Work out the finished part from the listing and answer in its coordinate system (mm). Face numbers are marked on the shaded views. A direction names the side the tool comes from. Round coordinates to 2 decimals unless told otherwise and drop trailing zeros. Order: outer loops, then holes, each group sorted by start corner. A loop starts at its lowest first (then second) coordinate and runs counter-clockwise, first axis right, second up. Notation, with made-up numbers: M 33,15 L 47,15 A30 cw 47,45 Z; hole C 5,-20.75 d3. An arc over 180 degrees is marked long. Answer as a JSON object with one key per item and string values. Group by question number.
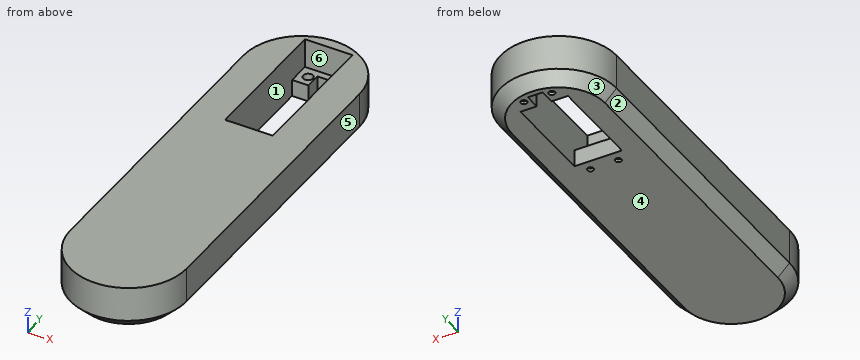
from build123d import *

# Parameters (mm, degrees)
BOSS_EXTRUDE1_DEPTH = 10
CHAMFER1_SIZE       = 5
CUT_EXTRUDE1_DEPTH  = 10.25
SKETCH5_W           = 6.4
SKETCH5_H           = 6.71
CUT_EXTRUDE2_DEPTH  = 24


with BuildPart() as part:
    # Sketch1 → Boss-Extrude1 (new, symmetric)
    with BuildSketch(Plane.XY):
        with BuildLine():
            Line((25, 130), (25, 0))
            ThreePointArc((25, 0), (0, -25), (-25, 0))
            Line((-25, 0), (-25, 130))
            ThreePointArc((-25, 130), (0, 155), (25, 130))
        make_face()
    extrude(amount=BOSS_EXTRUDE1_DEPTH, both=True)

    # Chamfer1
    chamfer1_edges = [part.edges().sort_by_distance(p)[0] for p in [
        (25, 65, -10),
        (0, -25, -10),
        (-25, 65, -10),
        (0, 155, -10),
    ]]
    chamfer(chamfer1_edges, length=CHAMFER1_SIZE)

    # Sketch3 → Cut-Extrude1 (cut, symmetric)
    with BuildSketch(Plane(origin=(0, 0, 0), x_dir=(0, 0, -1), z_dir=(1, 0, 0))):
        Polygon((2.7, 140.79), (2.7, 150.5), (-10, 150.5), (-10, 120.5), (10, 120.5), (10, 140.79), align=None)
    cut_extrude1 = extrude(amount=CUT_EXTRUDE1_DEPTH, both=True, mode=Mode.SUBTRACT)

    # Sketch4 → Cut-Revolve1 (revolve, cut)
    with BuildSketch(Plane(origin=(-6, 0, 0), x_dir=(0, 0, -1), z_dir=(1, 0, 0)), mode=Mode.PRIVATE) as cut_revolve1_sk:
        Polygon((2.7, 145.5), (12.7, 145.5), (12.7, 146.85), (8.7, 146.85), (8.7, 147.6), (2.7, 147.6), align=None)
    cut_revolve1 = revolve(cut_revolve1_sk.sketch.rotate(Axis((-6, 145.5, -58.145818423), (0, 0, 1)), 90), axis=Axis((-6, 145.5, -58.145818423), (0, 0, 1)), mode=Mode.SUBTRACT)

    # Mirror1: Cut-Revolve1 across plane
    add(cut_revolve1.mirror(Plane(origin=(0, 0, 0), x_dir=(0, 0, 1), z_dir=(1, 0, 0))), mode=Mode.SUBTRACT)

    # Mirror2: Cut-Extrude1, Cut-Revolve1 across plane
    add(cut_extrude1.mirror(Plane(origin=(-10.25, 120.5, -10), x_dir=(0, 0, 1), z_dir=(0, -1, 0))), mode=Mode.SUBTRACT)
    add(cut_revolve1.mirror(Plane(origin=(-10.25, 120.5, -10), x_dir=(0, 0, 1), z_dir=(0, -1, 0))), mode=Mode.SUBTRACT)

    # Mirror2 copy 1 sketch → Mirror2 copy 1 (revolve, cut)
    with BuildSketch(Plane(origin=(6, 241, 0), x_dir=(0, 0, -1), z_dir=(-1, 0, 0))):
        Polygon((2.7, 145.5), (12.7, 145.5), (12.7, 146.85), (8.7, 146.85), (8.7, 147.6), (2.7, 147.6), align=None)
    revolve(axis=Axis((6, 95.5, -58.145818423), (0, 0, 1)), mode=Mode.SUBTRACT)

    # Sketch5 → Cut-Extrude2 (cut)
    with BuildSketch(Plane.XY.offset(-2.7)):
        with Locations((0, 144.145)):
            Rectangle(SKETCH5_W, SKETCH5_H)
    extrude(amount=-CUT_EXTRUDE2_DEPTH, mode=Mode.SUBTRACT)


solid = part.part
Item 1: Each of these flat-tipped pins is pushed along its axis until it touches: pin 1 (8 mm diameter, centred on x = -4, z = -6, fed in from +Y); pin 2 (5.5 mm diameter, centred on x = 8, z = -7.5, fed in from -Y); pin 3 (5.5 mm diameter, centred on x = -7, z = -8, fed in from -Y). Where does it stop, or does it pass through?
Item 2: The mould has two halves that part along X. Classify the marked faces 3, 4, 5 and 6: +X half, -X half, draft (parallel to the pull), parting line (faces both ways), or undercut.
Item 3: Consider L1, parallel to X at y = 145.5, z = -5.7; L2, parallel to Y at x = -6, z = -9.2; L3, parallel to Y at x = -6, z = -6. Determine where each line is inside the solid, lowest interval first.
Item 4: Find section B-B (z = 7.5). Give the vertices of the cut face in (x, y).
Item 5: A tool of negligible diameter and unlimited length cuts with its end or side. For the marked faces 1 and 2, from which of +Z, -Z, +X, -X, +Y, -Y can it reach the whole face along a straight path? Write none if from no direction.
Item 6: Find section C-C (y = 29). Give the vertices of the cut face in (x, z).
Item 7: Find section A-A (x = 0). Give the vertices of the cut face in (y, z), and give its area (3 significant figures).
Responses:
{
 "1": {"pin 1": "stops at y = 155", "pin 2": "stops at y = -24.04", "pin 3": "stops at y = -23.84"},
 "2": {"face 3": "parting line", "face 4": "draft", "face 5": "+X half", "face 6": "undercut"},
 "3": {"L1": "x = -18.71 to -8.1, -3.9 to -3.2, 3.2 to 3.9, 8.1 to 18.71", "L2": "y = -19.92 to 94.15, 96.85 to 100.21, 140.79 to 144.15, 146.85 to 149.92", "L3": "y = -23.24 to 93.4, 97.6 to 100.21, 140.79 to 143.4, 147.6 to 153.24"},
 "4": {"outline": "M -25,0 A25 ccw 25,0 L 25,130 A25 ccw -25,130 Z; hole M -10.25,90.5 L 10.25,90.5 L 10.25,150.5 L -10.25,150.5 Z"},
 "5": {"face 1": "+Z", "face 2": "-Z, -X, +Y, -Y"},
 "6": {"outline": "M -25,-5 L -20,-10 L 20,-10 L 25,-5 L 25,10 L -25,10 Z"},
 "7": {"outline": "M -25,-5 L -20,-10 L 100.21,-10 L 100.21,-2.7 L 90.5,-2.7 L 90.5,10 L -25,10 Z; M 147.5,-10 L 150,-10 L 155,-5 L 155,10 L 150.5,10 L 150.5,-2.7 L 147.5,-2.7 Z", "area": "2,470 mm^2"}
}
